Geometry check sheet. Reference: the model listing, model coordinates, mm. A direction names the side the tool comes from. Coordinates: 2 decimals unless noted, no trailing zeros. Loops run counter-clockwise (first coordinate to the right, second up) from the corner with the lowest first, then second, coordinate; pieces in that order, holes last. Notation, with made-up numbers: (-21, 54.5) - (18, 54.5) arc R26 cw to (18, 75.5) - close; hole circle Ø7 at (-4.5, 8). An arc over 180 degrees is marked (long way). Write each question's results on one line, items separated by ' | '. Start each with the question number.
(1) Sectioned sample at B-B (z = 8.5). Enter the section's corners in (x, y).
(2) Sectioned sample at C-C (y = 29). Enter the section's corners in (x, z), plus the area to 3 significant figures.
(3) Material ranges on probe 1 along X at (y, z) = (40, 6.25); probe 2 along Y at (x, z) = (79.5, 9.25); probe 3 along Z at (x, y) = (14.5, 17), recorded low to high.
(4) Sectioned sample at A-A (x = 35.5). Enter the section's corners in (y, z), plus the area to 3 significant figures.
(5) Go/stop test with flat-tipped pins: pin 1 Ø20 at (x, y) = (58, 46.5) entering from +Z; pin 2 Ø12 at (x, y) = (18, 36.5) entering from -Z; pin 3 Ø4.5 at (y, z) = (34.28, 4.53) entering from +X. Record where each tip stops, or that it passes through.
(6) Access from +Z, -Z, +X, -X, +Y, -Y to the whole of each face (thin tool, end or side, straight path). Record for faces 4 (the face through (10, 43, 1)), 5 (the face through (2, 35, 7)), 6 (the face through (41, 0, 5)).
(7) Mould release check, pull along Z, two halves, no side actions. Record for faces 1 (the face through (0, 35, 5)), 2 (the face through (82.014, 35.97, 6.375)), 3 (the face through (38, 1, 10)): pulls with the +Z half, pulls with the -Z half, needs draft (parallel to the pull), parting line crosses it, or undercut.
(8) Sectioned sample at D-D (y = 15). Enter the section's corners in (x, z), plus the area to 3 significant figures.
from build123d import *

# Parameters (mm, degrees)
SKETCH1_W           = 83
SKETCH1_H           = 70
BOSS_EXTRUDE1_DEPTH = 10
SKETCH3_W           = 79
SKETCH3_H           = 66
CUT_EXTRUDE1_DEPTH  = 7
SKETCH4_W           = 30
SKETCH4_H           = 30
CUT_EXTRUDE2_DEPTH  = 7
SKETCH5_R           = 2.5
CUT_EXTRUDE3_DEPTH  = 2


with BuildPart() as part:
    # Sketch1 → Boss-Extrude1 (new body)
    with BuildSketch(Plane.XY):
        with Locations((41.5, 35)):
            Rectangle(SKETCH1_W, SKETCH1_H)
    extrude(amount=BOSS_EXTRUDE1_DEPTH)

    # Sketch3 → Cut-Extrude1 (cut)
    with BuildSketch(Plane.XY.offset(10)):
        with Locations((41.5, 35)):
            Rectangle(SKETCH3_W, SKETCH3_H)
    extrude(amount=-CUT_EXTRUDE1_DEPTH, mode=Mode.SUBTRACT)

    # Sketch4 → Cut-Extrude2 (cut)
    with BuildSketch(Plane(origin=(0, 0, 0), x_dir=(-1, 0, 0), z_dir=(0, 0, -1))):
        with Locations((-25, 43)):
            Rectangle(SKETCH4_W, SKETCH4_H)
    extrude(amount=-CUT_EXTRUDE2_DEPTH, mode=Mode.SUBTRACT)

    # Sketch5 → Cut-Extrude3 (cut)
    with BuildSketch(Plane(origin=(83, 0, 0), x_dir=(0, 0, -1), z_dir=(1, 0, 0))):
        with Locations((-4.532050628, 34.280077889)):
            Circle(SKETCH5_R)
    extrude(amount=-CUT_EXTRUDE3_DEPTH, mode=Mode.SUBTRACT)


solid = part.part
Outcome:
1) outline: (0, 0) - (83, 0) - (83, 70) - (0, 70) - close; hole (2, 2) - (81, 2) - (81, 68) - (2, 68) - close
2) outline: (0, 0) - (10, 0) - (10, 3) - (2, 3) - (2, 10) - (0, 10) - close; (40, 0) - (83, 0) - (83, 10) - (81, 10) - (81, 3) - (40, 3) - close | area: 187 mm2
3) probe 1: x = 0 to 2, 81 to 83 | probe 2: y = 0 to 2, 68 to 70 | probe 3: z = 0 to 3
4) outline: (0, 0) - (28, 0) - (28, 3) - (2, 3) - (2, 10) - (0, 10) - close; (58, 0) - (70, 0) - (70, 10) - (68, 10) - (68, 3) - (58, 3) - close | area: 148 mm2
5) pin 1: stops at z = 3 | pin 2: passes through | pin 3: stops at x = 81
6) face 4: +Z, -Z | face 5: +Z | face 6: +Z, -Z, +X, -X, -Y
7) face 1: needs draft | face 2: undercut | face 3: pulls with the +Z half
8) outline: (0, 0) - (83, 0) - (83, 10) - (81, 10) - (81, 3) - (2, 3) - (2, 10) - (0, 10) - close | area: 277 mm2
